```python
from build123d import *

# Parameters (mm, degrees)
SKETCH2_W               = 19.05
SKETCH2_H               = 31.75
BOSS_EXTRUDE1_DEPTH     = 76.2
SKETCH3_W               = 25.4
SKETCH3_H               = 50.8
BOSS_EXTRUDE2_DEPTH     = 63.5
FILLET1_R               = 6.35
SKETCH4_R               = 12.7
CUT_EXTRUDE1_DEPTH      = 145.244271983
CUT_EXTRUDE2_REACH      = 151.191
CUT_EXTRUDE2_END_RADIUS = 12.7
SKETCH5_R               = 2.4892
CUT_EXTRUDE3_REACH      = 145.719
SKETCH6_R               = 2.4892


with BuildPart() as part:
    # Sketch2 → Boss-Extrude1 (new body)
    with BuildSketch(Plane(origin=(0, 0, 0), x_dir=(1, 0, 0), z_dir=(0, 1, 0))):
        Rectangle(SKETCH2_W, SKETCH2_H)
    extrude(amount=BOSS_EXTRUDE1_DEPTH)

    # Sketch3 → Boss-Extrude2 (add)
    with BuildSketch(Plane(origin=(0, 76.2, 0), x_dir=(1, 0, 0), z_dir=(0, 1, 0))):
        Rectangle(SKETCH3_W, SKETCH3_H)
    extrude(amount=BOSS_EXTRUDE2_DEPTH)

    # Fillet1
    fillet1_edges = [part.edges().sort_by_distance(p)[0] for p in [
        (0, 139.7, -25.4),
        (0, 139.7, 25.4),
    ]]
    fillet(fillet1_edges, radius=FILLET1_R)

    # Sketch4 → Cut-Extrude1 (cut, through all)
    with BuildSketch(Plane(origin=(12.7, 0, 0), x_dir=(0, 0, -1), z_dir=(1, 0, 0))):
        with Locations((0, 120.65)):
            Circle(SKETCH4_R)
    extrude(amount=-CUT_EXTRUDE1_DEPTH, mode=Mode.SUBTRACT)

    # Cut-Extrude2: up to this cylinder (the profile starts outside it)
    cut_extrude2_end = Plane(origin=(0, 120.65, 0), z_dir=(1, 0, 0)) * Cylinder(CUT_EXTRUDE2_END_RADIUS, 328.782, mode=Mode.PRIVATE)
    # Sketch5 → Cut-Extrude2 (cut, up to the surface)
    with BuildSketch(Plane(origin=(0, 0, -25.4), x_dir=(-1, 0, 0), z_dir=(0, 0, -1)), mode=Mode.PRIVATE) as cut_extrude2_sk1:
        with Locations((0, 120.65)):
            Circle(SKETCH5_R)
    cut_extrude2_tool1 = extrude(cut_extrude2_sk1.sketch, amount=-CUT_EXTRUDE2_REACH, mode=Mode.PRIVATE) - cut_extrude2_end
    add(cut_extrude2_tool1.solids().sort_by_distance((0, 120.65, -25.4))[0], mode=Mode.SUBTRACT)

    # Sketch6 → Cut-Extrude3 (cut, up to next)
    with BuildSketch(Plane.ZY.offset(9.525), mode=Mode.PRIVATE) as cut_extrude3_sk1:
        with Locations((0, 25.4)):
            Circle(SKETCH6_R)
    cut_extrude3_tool1 = extrude(cut_extrude3_sk1.sketch, amount=-CUT_EXTRUDE3_REACH, mode=Mode.PRIVATE) & part.part
    # Sketch6 → Cut-Extrude3 (cut, up to next)
    with BuildSketch(Plane.ZY.offset(9.525), mode=Mode.PRIVATE) as cut_extrude3_sk2:
        with Locations((0, 50.8)):
            Circle(SKETCH6_R)
    cut_extrude3_tool2 = extrude(cut_extrude3_sk2.sketch, amount=-CUT_EXTRUDE3_REACH, mode=Mode.PRIVATE) & part.part
    add(cut_extrude3_tool1.solids().sort_by_distance((-9.525, 25.4, 0))[0], mode=Mode.SUBTRACT)
    add(cut_extrude3_tool2.solids().sort_by_distance((-9.525, 50.8, 0))[0], mode=Mode.SUBTRACT)


solid = part.part
```
Could you check a few things on this model? Use its own coordinates, in mm. A direction names the side the tool comes from. Coordinates: 2 decimals unless noted, no trailing zeros. Loops run counter-clockwise (first coordinate to the right, second up) from the corner with the lowest first, then second, coordinate; pieces in that order, holes last. Notation, with made-up numbers: M 89.5,3.5 L 95.5,3.5 A15 ccw 95.5,14.5 Z; hole C 54.25,44.25 d3. An arc over 180 degrees is marked long. Put each result on its own line as item: value. Start each with the question number.
(1) Thinking about a two-plate mould opening in Y: for faces 6 (the face through (0.178, 109.383, -5.86)), 7 (the face through (0, 139.7, 0)), 8 (the face through (11, 76.2, 0)), 9 (the face through (9.525, 38, 0)), which applies, pulls with the +Y half, pulls with the -Y half, needs draft (parallel to the pull), parting line crosses it, or undercut?
(2) Suppose I cut it at B-B on x = 0. Please give me the cut outline in (y, z) (3 decimals).
(3) Suppose I cut it at D-D on x = 6.5. Please give me the cut outline in (y, z) (3 decimals).
(4) Suppose I cut it at C-C on z = 0. Please give me the cut outline in (x, y) (3 decimals), then the cut area to 3 significant figures.
(5) Will these pins go through, and if not, where does the flat tip stop? P1, Ø3, axis at x = 8.5, y = 29.5, coming from the -Z side (3 decimals); P2, Ø3, axis at y = 25.4, z = 0, coming from the +X side; P3, Ø1, axis at y = 63.5, z = 7.5, coming from the +X side (3 decimals); P4, Ø16, axis at y = 49.5, z = 5, coming from the -X side (3 decimals).
(6) I need wall thicknesses on line 1 (Y direction, x = 0.5, z = 0); line 2 (Z direction, x = -3, y = 19.5) (3 decimals); line 3 (X direction, y = 43, z = 9) (3 decimals). Which ranges of each line are inside material? Lowest first, please. Write a range as from..to.
(7) Suppose I cut it at A-A on y = 50.8. Please give me the cut outline in (x, z) (3 decimals).
(8) For faces 1 (the face through (0, 104, -25.4)), 2 (the face through (-9.525, 38, 0)), 3 (the face through (0.54, 118.22, -19.02)), 4 (the face through (0, 38, 15.875)), 5 (the face through (0, 38, -15.875)), which set-ups out of +Z, -Z, +X, -X, +Y, -Y let a thin tool reach every point of the face, with its end or its side?
Solutions:
1. face 6: undercut
1. face 7: pulls with the +Y half
1. face 8: pulls with the -Y half
1. face 9: needs draft
2. outline: M 0,-15.875 L 76.2,-15.875 L 76.2,-25.4 L 118.161,-25.4 L 118.161,-12.454 A12.7 cw long 123.139,-12.454 L 123.139,-25.4 L 133.35,-25.4 A6.35 ccw 139.7,-19.05 L 139.7,19.05 A6.35 ccw 133.35,25.4 L 76.2,25.4 L 76.2,15.875 L 0,15.875 Z; hole C 25.4,0 d4.978; hole C 50.8,0 d4.978
3. outline: M 0,-15.875 L 76.2,-15.875 L 76.2,-25.4 L 133.35,-25.4 A6.35 ccw 139.7,-19.05 L 139.7,19.05 A6.35 ccw 133.35,25.4 L 76.2,25.4 L 76.2,15.875 L 0,15.875 Z; hole C 25.4,0 d4.978; hole C 50.8,0 d4.978; hole C 120.65,0 d25.4
4. outline: M -12.7,76.2 L -9.525,76.2 L -9.525,53.289 L 9.525,53.289 L 9.525,76.2 L 12.7,76.2 L 12.7,107.95 L -12.7,107.95 Z; M -12.7,133.35 L 12.7,133.35 L 12.7,139.7 L -12.7,139.7 Z; M -9.525,0 L 9.525,0 L 9.525,22.911 L -9.525,22.911 Z; M -9.525,27.889 L 9.525,27.889 L 9.525,48.311 L -9.525,48.311 Z
4. area: 2,230 mm2
5. P1: stops at z = -15.875
5. P2: passes through
5. P3: stops at x = 9.525
5. P4: stops at x = -9.525
6. line 1: y = 0..22.91, 27.89..48.31, 53.29..107.95, 133.35..139.7
6. line 2: z = -15.875..15.875
6. line 3: x = -9.525..9.525
7. outline: M -9.525,-15.875 L 9.525,-15.875 L 9.525,-2.489 L -9.525,-2.489 Z; M -9.525,2.489 L 9.525,2.489 L 9.525,15.875 L -9.525,15.875 Z
8. face 1: -Z, +X, -X, +Y, -Y
8. face 2: +Z, -Z, -X, -Y
8. face 3: -Z
8. face 4: +Z, +X, -X, -Y
8. face 5: -Z, +X, -X, -Y
